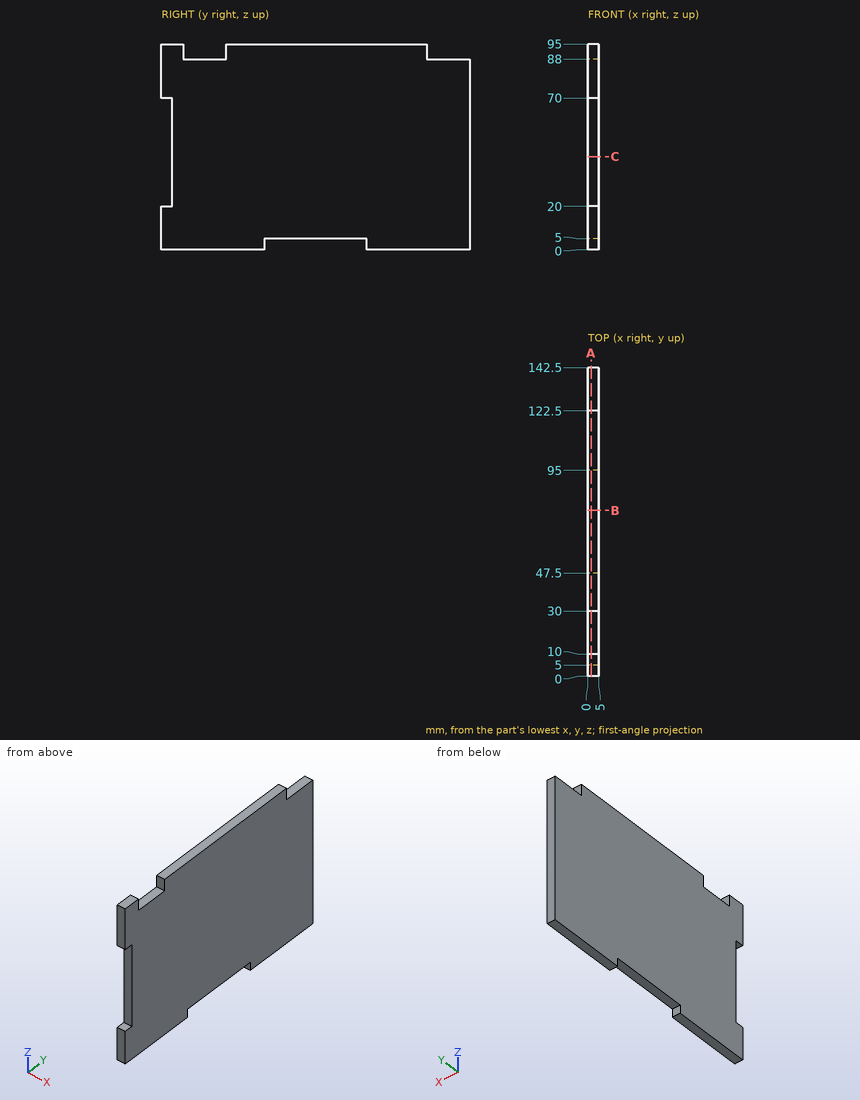
Print and shaded views of the part. All mm, measured from the part's lowest x, y and z. Coordinates: 2 decimals unless noted, no trailing zeros. Loops run counter-clockwise (first coordinate to the right, second up) from the corner with the lowest first, then second, coordinate; pieces in that order, holes last. Notation, with made-up numbers: (55, 12.5) -> (66, 12.5) arc R11 cw to (66, 28.5) -> close; hole circle Ø8 at (4.5, 86.25). An arc over 180 degrees is marked (long way). Use a Markdown table: item, result. Add a question column.
Item 1: Probe probe 1 along Y at (x, z) = (2.6, 91.5); probe 2 along Z at (x, y) = (2.5, 17.5); probe 3 along Y at (x, z) = (0.6, 44). List the from-to ranges inside material, lowest first.
Item 2: Band-saw the part on C-C on z = 43. Write the cut outline in (x, y), plus the area to 4 significant figures.
Item 3: Band-saw the part on A-A on x = 1.55. Write the cut outline in (y, z).
Item 4: Band-saw the part on B-B on y = 76.5. Write the cut outline in (x, z).
Item 5: Flat gauge pins, fed straight in: P1, Ø1.5, axis at x = 0.5, y = 17, coming from the -Z side; P2, Ø1.5, axis at x = 3.5, y = 18.5, coming from the +Z side; P3, Ø2.5, axis at x = 2.5, y = 76, coming from the -Z side. Where does each tip first touch, or does it go through?
Geometry says:
| question | item | result |
|---|---|---|
| 1 | probe 1 | 0 to 10, 30 to 122.5 |
| 1 | probe 2 | 0 to 88 |
| 1 | probe 3 | 5 to 142.5 |
| 2 | outline | (0, 5) -> (5, 5) -> (5, 142.5) -> (0, 142.5) -> close |
| 2 | area | 687.5 mm² |
| 3 | outline | (0, 0) -> (47.5, 0) -> (47.5, 5) -> (95, 5) -> (95, 0) -> (142.5, 0) -> (142.5, 88) -> (122.5, 88) -> (122.5, 95) -> (30, 95) -> (30, 88) -> (10, 88) -> (10, 95) -> (0, 95) -> (0, 70) -> (5, 70) -> (5, 20) -> (0, 20) -> close |
| 4 | outline | (0, 5) -> (5, 5) -> (5, 95) -> (0, 95) -> close |
| 5 | P1 | z = 0 |
| 5 | P2 | z = 88 |
| 5 | P3 | z = 5 |
